Geometry: see drawing. Coordinates: mm, zero at the bounding-box minimum. A direction names the side the tool comes from. Round coordinates to 2 decimals unless told otherwise and drop trailing zeros. Loops run counter-clockwise (first coordinate to the right, second up) from the corner with the lowest first, then second, coordinate; pieces in that order, holes last.
(1) Draft query along Y for the marked faces 3, 4 and 5. Return one class per face: released by +Y, released by -Y, zero draft, split by the parting line, or undercut.
(2) Cut plane B-B, the plane z = 2.5. Output: boundary loops of the cut face in (x, y) (1 decimal).
(3) Line query: line 1 (Z direction, x = 2.05, y = 0.4); line 2 (X direction, y = 2, z = 7); line 3 (Z direction, x = 1.15, y = 1.85) (1 decimal). Output: solid intervals per line, ascending.
(4) Access query for the marked faces 1 and 2. Directions: +Z, -Z, +X, -X, +Y, -Y. A direction counts if a zero-diameter tool reaches every point of the face in a straight line with its end or side. Return the directions, or none.
(5) First-contact query: pin 1 Ø2 at (y, z) = (1, 7) entering from +X (3 decimals); pin 2 Ø1.5 at (x, z) = (1, 5.5) entering from +Y; pin 3 Ø1.6 at (x, y) = (1.5, 2) entering from -Z. Flat tips, straight axial feed; report the tip coordinate or a pass-through.
(6) Cut plane A-A, the plane z = 1.5. Output: boundary loops of the cut face in (x, y) (1 decimal).
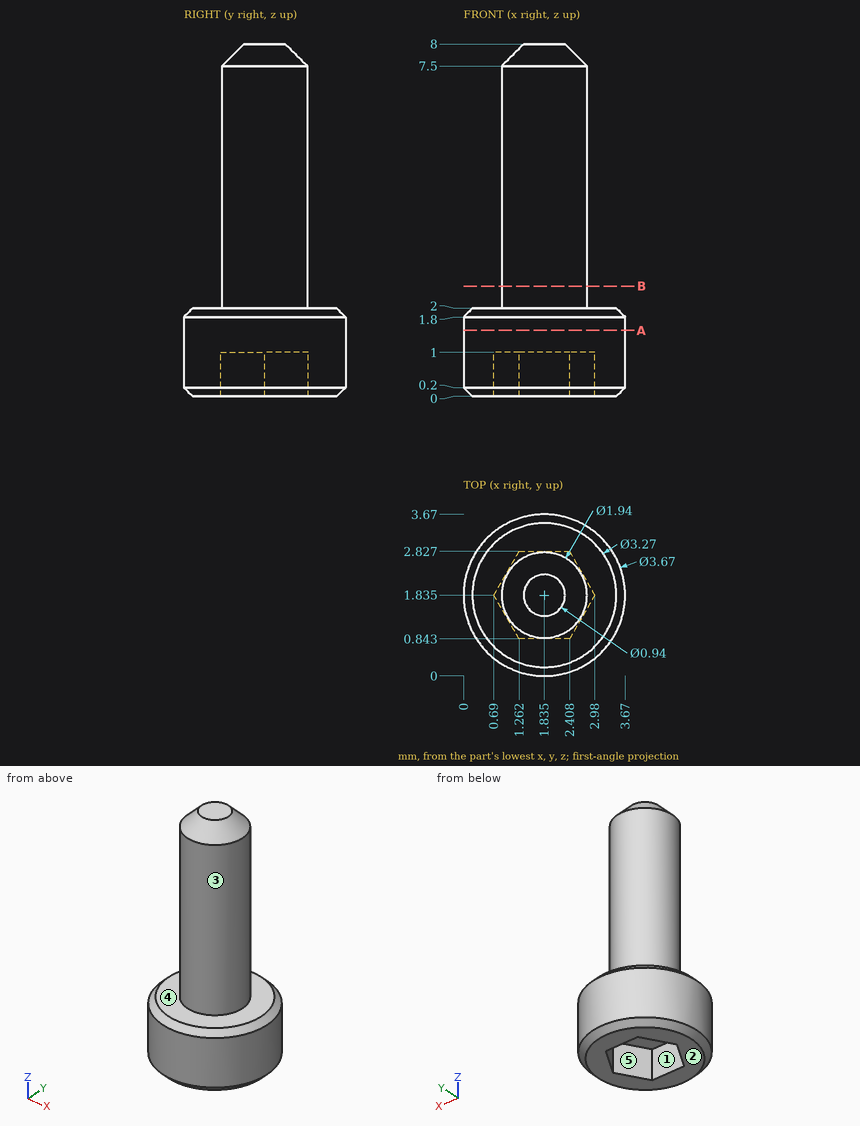
Reported:
1. face 3: split by the parting line
1. face 4: zero draft
1. face 5: undercut
2. outline: circle Ø1.9 at (1.8, 1.8)
3. line 1: z = 0 to 2
3. line 2: x = 0.88 to 2.79
3. line 3: z = 1 to 7.8
4. face 1: -Z
4. face 2: -Z, +X, -X, +Y, -Y
5. pin 1: stops at x = 2.805
5. pin 2: stops at y = 2.8
5. pin 3: stops at z = 0
6. outline: circle Ø3.7 at (1.8, 1.8)
